Verification items for the finished model (mm, model axes). A direction names the side the tool comes from. Coordinates: 2 decimals unless noted, no trailing zeros. Order: outer loops, then holes, each group sorted by start corner. A loop starts at its lowest first (then second) coordinate and runs counter-clockwise, first axis right, second up. Notation, with made-up numbers: M -4,22 L 43,22 A24 cw 43,44 Z; hole C 62.5,-24 d4. An arc over 180 degrees is marked long. Return JSON: item names as keys, results as strings.
```python
from build123d import *

# Parameters (mm, degrees)
F1_DEPTH = 25


with BuildPart() as f1:
    # F0 (on Front) → F1 (new body)
    with BuildSketch(Plane.XZ):
        with BuildLine():
            ThreePointArc((28.481623, 6.237598), (27.602944, 8.358919), (25.481623, 9.237598))
            Line((25.481623, 9.237598), (18.819672, 9.237598))
            ThreePointArc((18.819672, 9.237598), (17.759012, 8.798258), (17.319672, 7.737598))
            Line((17.319672, 7.737598), (17.319672, -0.762402))
            Line((17.319672, -0.762402), (-26.034861, -6.459927))
            Line((-26.034861, -6.459927), (-26.034861, -12.899362))
            Line((-26.034861, -12.899362), (-40.034861, -12.899362))
            Line((-40.034861, -12.899362), (-40.034861, -8.299765))
            Line((-40.034861, -8.299765), (-73.418925, -12.687001))
            Line((-73.418925, -12.687001), (-73.730306, -12.727921))
            ThreePointArc((-73.730306, -12.727921), (-74.662506, -13.225985), (-75.034861, -14.215134))
            Line((-75.034861, -14.215134), (-75.034861, -43.585033))
            ThreePointArc((-75.034861, -43.585033), (-74.663044, -44.573569), (-73.731923, -45.072032))
            Line((-73.731923, -45.072032), (-40.034861, -49.537685))
            Line((-40.034861, -49.537685), (-40.034861, -44.899362))
            Line((-40.034861, -44.899362), (-26.034861, -44.899362))
            Line((-26.034861, -44.899362), (-26.034861, -51.393015))
            Line((-26.034861, -51.393015), (14.481623, -56.762402))
            Line((14.481623, -56.762402), (14.481623, -65.262402))
            ThreePointArc((14.481623, -65.262402), (14.920963, -66.323062), (15.981623, -66.762402))
            Line((15.981623, -66.762402), (25.481623, -66.762402))
            ThreePointArc((25.481623, -66.762402), (27.602944, -65.883722), (28.481623, -63.762402))
            Line((28.481623, -63.762402), (28.481623, 6.237598))
        make_face()
    extrude(amount=F1_DEPTH)


solid = f1.part
```
Q1. Go/stop test with flat-tipped pins: pin 1 (5 mm diameter, centred on x = -41, y = -14.5, fed in from -Z); pin 2 (2.5 mm diameter, centred on y = -8, z = 4, fed in from -X); pin 3 (7 mm diameter, centred on x = -32.5, y = -16, fed in from -Z). Record where each tip stops, or that it passes through.
Values:
{"pin 1": "z = -49.54", "pin 2": "x = 17.32", "pin 3": "z = -44.9"}
Q2. Tool access check on faces 1 (the face through (17.32, -12, 4)), 2 (the face through (-40.035, -12, -11)), 3 (the face through (-33, -12, -44.899)). Record the directions out of +Z, -Z, +X, -X, +Y, -Y that give a thin tool (end or side, any length) a straight path to the whole face; none if there is none.
Values:
{"face 1": "+Z, -X, +Y, -Y", "face 2": "+Z, +Y, -Y", "face 3": "-Z, +Y, -Y"}
Q3. Cross-section at B-B, the plane z = -60. Record the boundary of the cut face in (x, y), and give its area (3 significant figures).
Values:
{"outline": "M 14.48,-25 L 28.48,-25 L 28.48,0 L 14.48,0 Z", "area": "350 mm^2"}
Q4. Material ranges on line 1 along Z through (x, y) = (-36.5, -18.25); line 2 along X through (y, z) = (-10.25, -62); line 3 along Z through (x, y) = (7, -2.5), recorded low to high.
Values:
{"line 1": "-44.9 to -12.9", "line 2": "14.48 to 28.48", "line 3": "-55.77 to -2.12"}
Q5. Cross-section at C-C, the plane x = 8. Record the boundary of the cut face in (y, z).
Values:
{"outline": "M -25,-55.9 L 0,-55.9 L 0,-1.99 L -25,-1.99 Z"}
Q6. Cross-section at A-A, the plane y = -14. Record the boundary of the cut face in (x, z).
Values:
{"outline": "M -75.03,-43.59 A1.5 ccw -73.73,-45.07 L -40.03,-49.54 L -40.03,-44.9 L -26.03,-44.9 L -26.03,-51.39 L 14.48,-56.76 L 14.48,-65.26 A1.5 ccw 15.98,-66.76 L 25.48,-66.76 A3 ccw 28.48,-63.76 L 28.48,6.24 A3 ccw 25.48,9.24 L 18.82,9.24 A1.5 ccw 17.32,7.74 L 17.32,-0.76 L -26.03,-6.46 L -26.03,-12.9 L -40.03,-12.9 L -40.03,-8.3 L -73.42,-12.69 L -73.73,-12.73 A1.5 ccw -75.03,-14.22 Z"}
